Source: three-view drawing plus pictorial views. Frame: mm from the lowest corner of the part. Coordinates: 2 decimals unless noted, no trailing zeros. Order: outer loops, then holes, each group sorted by start corner. A loop starts at its lowest first (then second) coordinate and runs counter-clockwise, first axis right, second up. Notation, with made-up numbers: M 13,56 L 65,56 A25 cw 65,85 Z; hole C 50,16.5 d6. An arc over 180 degrees is marked long. Use CSV: the item, a comma, the result in double quotes. Start each with the question number.
Q1. Ray query, probe 1 along Z at (x, y) = (2.9, 46.5); probe 2 along Z at (x, y) = (2.9, 12.5); probe 3 along Y at (x, z) = (1.05, 53). Return the intervals inside material, ascending.
Q2. Section query B-B, the plane z = 42. Output: boundary loops of the cut face in (x, y).
Q3. Section query C-C, the plane y = 17. Output: boundary loops of the cut face in (x, z).
Q4. First-contact query: P1, Ø12, axis at y = 8, z = 8, coming from the -X side; P2, Ø12, axis at y = 30, z = 24.5, coming from the +X side; P3, Ø1.5, axis at x = 2.5, z = 3, coming from the -Y side; P4, Ø0.9, axis at y = 3, z = 3, coming from the -X side. Flat tips, straight axial feed; report the tip coordinate or a pass-through.
Q5. Section query D-D, the plane x = 2. State how many separate pieces and enclosed holes the cut face has, and give its area (3 significant figures).
Q6. Section query A-A, the plane y = 46.5. Output: boundary loops of the cut face in (x, z).
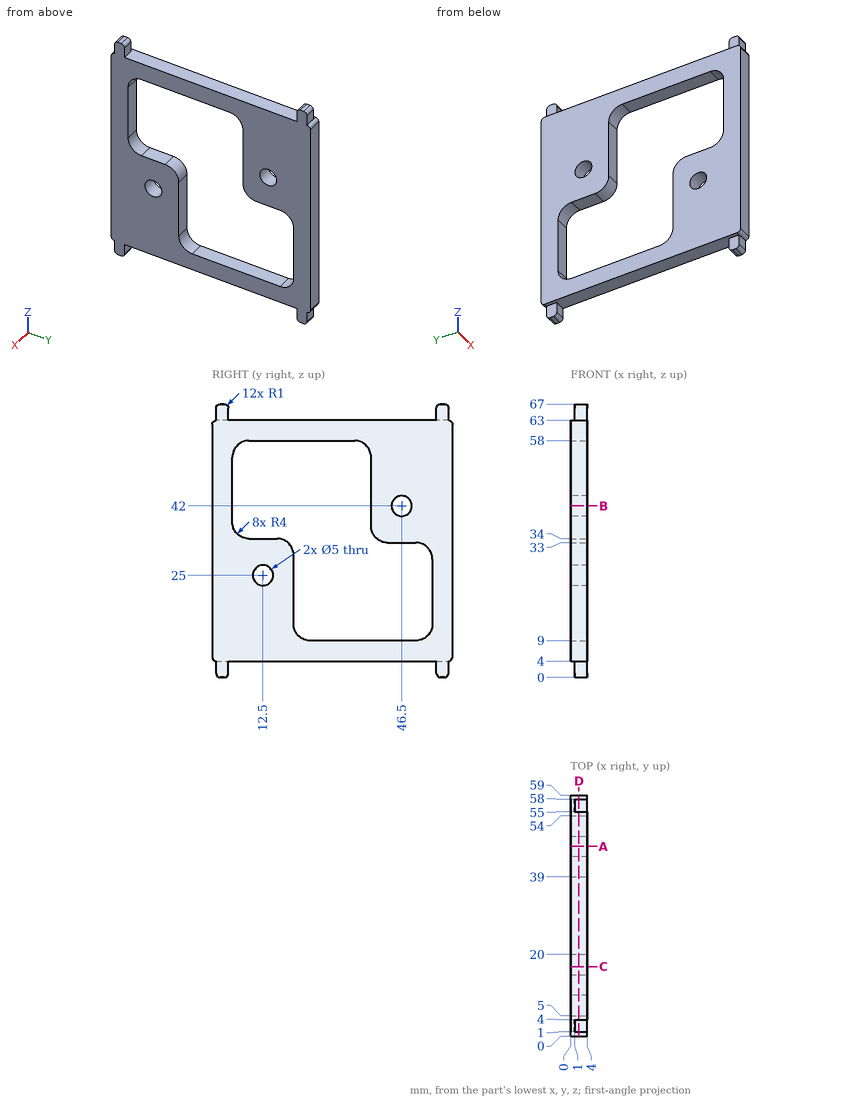
Responses:
1,probe 1,"z = 4 to 9, 33 to 39.5, 44.5 to 63"
1,probe 2,"z = 4 to 22.5, 27.5 to 34, 58 to 63"
1,probe 3,"y = 0 to 5, 39 to 59"
2,outline,"M 0,0 L 4,0 L 4,5 L 0,5 Z; M 0,39 L 4,39 L 4,44 L 0,44 Z; M 0,49 L 4,49 L 4,59 L 0,59 Z"
3,outline,"M 0,4 L 4,4 L 4,33.87 L 0,33.87 Z; M 0,58 L 4,58 L 4,63 L 0,63 Z"
4,P1,"stops at x = 0"
4,P2,"passes through"
4,P3,"stops at y = 1"
4,P4,"stops at x = 1"
5,separate pieces,"1"
5,enclosed holes,"3"
5,area,"1,850 mm²"
6,outline,"M 0,4 L 4,4 L 4,9 L 0,9 Z; M 0,33 L 4,33 L 4,39.5 L 0,39.5 Z; M 0,44.5 L 4,44.5 L 4,63 L 0,63 Z"
